```python
from build123d import *

# Parameters (mm, degrees)
SKETCH1_W               = 56
SKETCH1_H               = 56
BOSS_EXTRUDE1_DEPTH     = 5
SKETCH2_R               = 8
BOSS_EXTRUDE2_DEPTH     = 15
SKETCH4_R               = 19
CUT_EXTRUDE2_DEPTH      = 2
CUT_EXTRUDE3_DEPTH      = 44.497126342
CUT_EXTRUDE3_DEPTH_BACK = 44.497126342
SKETCH5_R               = 7.5
SKETCH6_R               = 4
CUT_EXTRUDE4_DEPTH      = 15


with BuildPart() as part:
    # Sketch1 → Boss-Extrude1 (new body)
    with BuildSketch(Plane(origin=(0, 0, 0), x_dir=(1, 0, 0), z_dir=(0, 1, 0))):
        Rectangle(SKETCH1_W, SKETCH1_H)
    extrude(amount=BOSS_EXTRUDE1_DEPTH)

    # Sketch2 → Boss-Extrude2 (add)
    with BuildSketch(Plane(origin=(0, 5, 0), x_dir=(1, 0, 0), z_dir=(0, 1, 0))):
        with Locations(Location((15, 15, 0), (0, 0, 90))):
            Circle(SKETCH2_R)
    extrude(amount=BOSS_EXTRUDE2_DEPTH)

    # Sketch4 → Cut-Extrude2 (cut)
    with BuildSketch(Plane.XZ):
        with Locations(Location((0, 0, 0), (0, 0, 270))):
            Circle(SKETCH4_R)
    extrude(amount=-CUT_EXTRUDE2_DEPTH, mode=Mode.SUBTRACT)

    # Sketch5 → Cut-Extrude3 (cut, two sides: drawn at the far end of the back side and taken through both)
    with BuildSketch(Plane.XZ.offset(-2).offset(-CUT_EXTRUDE3_DEPTH_BACK)):
        with Locations(Location((0, 0, 0), (0, 0, 270))):
            Circle(SKETCH5_R)
    extrude(amount=CUT_EXTRUDE3_DEPTH + CUT_EXTRUDE3_DEPTH_BACK, mode=Mode.SUBTRACT)

    # Sketch6 → Cut-Extrude4 (cut)
    with BuildSketch(Plane(origin=(0, 20, 0), x_dir=(1, 0, 0), z_dir=(0, 1, 0))):
        with Locations(Location((15, 15, 0), (0, 0, 270))):
            Circle(SKETCH6_R)
    extrude(amount=-CUT_EXTRUDE4_DEPTH, mode=Mode.SUBTRACT)


solid = part.part
```
The listing builds one solid part. Answer for the finished solid, in the listing's coordinates (mm). A direction names the side the tool comes from. Give positions to 0.01 mm unless a question says otherwise; leave off trailing zeros. Write each loop counter-clockwise with the first axis right and the second up, starting at its lowest first coordinate (ties: lowest second). Pieces come first, ordered by that corner, then holes. Notation, with made-up numbers: (15.25, -10.5) -> (58.25, -10.5) arc R9 cw to (58.25, -0.5) -> close; hole circle Ø7 at (61, 38). An arc over 180 degrees is marked (long way). Write item = value, one per line. Start each with the question number.
1) Determine the mould class of faces 1 (the face through (0, 2, -28)), 2 (the face through (-11.56, 0.99, 15.08)), 3 (the face through (-28, 2, 0)), 4 (the face through (15, 5, -15)) for opening direction X: +X half, -X half, draft (parallel to the pull), parting line (faces both ways), or undercut.
2) Which of the six approach directions +Z, -Z, +X, -X, +Y, -Y give full straight-line access (tool end or side, diameter ignored) to faces 5 (the face through (0, 2, -8)), 6 (the face through (17, 20, -11)), 7 (the face through (17.7, 12.6, -17.95))?
3) The part is cut by section B-B, the plane x = 0. Determine the outline of the cut face in (y, z), and give its area (3 significant figures).
4) Each of these flat-tipped pins is pushed along its axis until it touches: pin 1 (5 mm diameter, centred on x = -3.5, z = -18.5, fed in from +Y); pin 2 (8 mm diameter, centred on y = 17.5, z = -16.5, fed in from -X); pin 3 (9 mm diameter, centred on x = 0, z = 0, fed in from +Y). Where does it stop, or does it pass through?
5) Straight lines are drawn through the part: line 1 along X through (y, z) = (16.75, -15); line 2 along X through (y, z) = (3.5, 0). For each, find the intervals that lie inside material, in ascending order.
6) The part is cut by section C-C, the plane y = 5.75. Determine the outline of the cut face in (x, z).
7) The part is cut by section D-D, the plane z = -15. Determine the outline of the cut face in (x, y).
8) The part is cut by section A-A, the plane z = 0. Determine the outline of the cut face in (x, y), and give its area (3 significant figures).
Solutions:
q1.face_1 = draft
q1.face_2 = undercut
q1.face_3 = -X half
q1.face_4 = undercut
q2.face_5 = -Y
q2.face_6 = +Z, -Z, +X, -X, +Y
q2.face_7 = +Y
q3.outline = (0, -28) -> (5, -28) -> (5, -7.5) -> (2, -7.5) -> (2, -19) -> (0, -19) -> close; (0, 19) -> (2, 19) -> (2, 7.5) -> (5, 7.5) -> (5, 28) -> (0, 28) -> close
q3.area = 159 mm²
q4.pin_1 = 5
q4.pin_2 = 7
q4.pin_3 = through
q5.line_1 = 7 to 11, 19 to 23
q5.line_2 = -28 to -7.5, 7.5 to 28
q6.outline = circle Ø16 at (15, -15); hole circle Ø8 at (15, -15)
q7.outline = (-28, 0) -> (-11.66, 0) -> (-11.66, 2) -> (11.66, 2) -> (11.66, 0) -> (28, 0) -> (28, 5) -> (23, 5) -> (23, 20) -> (19, 20) -> (19, 5) -> (11, 5) -> (11, 20) -> (7, 20) -> (7, 5) -> (-28, 5) -> close
q8.outline = (-28, 0) -> (-19, 0) -> (-19, 2) -> (-7.5, 2) -> (-7.5, 5) -> (-28, 5) -> close; (7.5, 2) -> (19, 2) -> (19, 0) -> (28, 0) -> (28, 5) -> (7.5, 5) -> close
q8.area = 159 mm²
